The drawing under review shows one solid part. Ordinate dimensions are in mm from its lowest x, y, z. A direction names the side the tool comes from. Coordinates: 2 decimals unless noted, no trailing zeros. Loops run counter-clockwise (first coordinate to the right, second up) from the corner with the lowest first, then second, coordinate; pieces in that order, holes last. Notation, with made-up numbers: (-5.5, 74.25) - (25.5, 74.25) arc R22 ccw to (25.5, 87.25) - close; hole circle Ø4 at (-19, 47.5). An arc over 180 degrees is marked (long way). Answer as a JSON object with one key per item and string values. Group by question number.
Item 1: We need section B-B (x = 8). Give the boundary of the cut face in (y, z).
Item 2: To check wall thickness, follow line 1 (Y direction, x = 42, z = 27.75); line 2 (X direction, y = 20, z = 6.75); line 3 (Y direction, x = 33.5, z = 18.75). State the ranges of each line that lie inside material, in increasing order.
Item 3: We need section A-A (x = 25). Give the boundary of the cut face in (y, z).
Item 4: We need section C-C (y = 25). Give the boundary of the cut face in (x, z), then the cut area to 3 significant figures.
Item 5: Tool access review of the marked faces 1, 2, 3, 4 and 5: name each direction out of +Z, -Z, +X, -X, +Y, -Y from which nothing blocks a thin tool from reaching the whole face with its end or side.
Item 6: Clearance check with flat-ended pins moving along their axes: pin 1 (13 mm diameter, centred on y = 22, z = 14.5, fed in from +X); pin 2 (5.5 mm diameter, centred on x = 23.5, y = 12.5, fed in from +Z); pin 3 (0.8 mm diameter, centred on x = 0.5, y = 25, fed in from +Z); pin 4 (1 mm diameter, centred on x = 42.5, z = 11, fed in from -Y). State where each tip first meets the part, or that it passes through.
Item 7: We need section D-D (z = 22.25). Give the boundary of the cut face in (x, y).
Item 8: Mouldability with a two-part tool opening along X and no side actions: class the marked faces 6, 7 and 8 as released by +X, released by -X, zero draft, split by the parting line, or undercut.
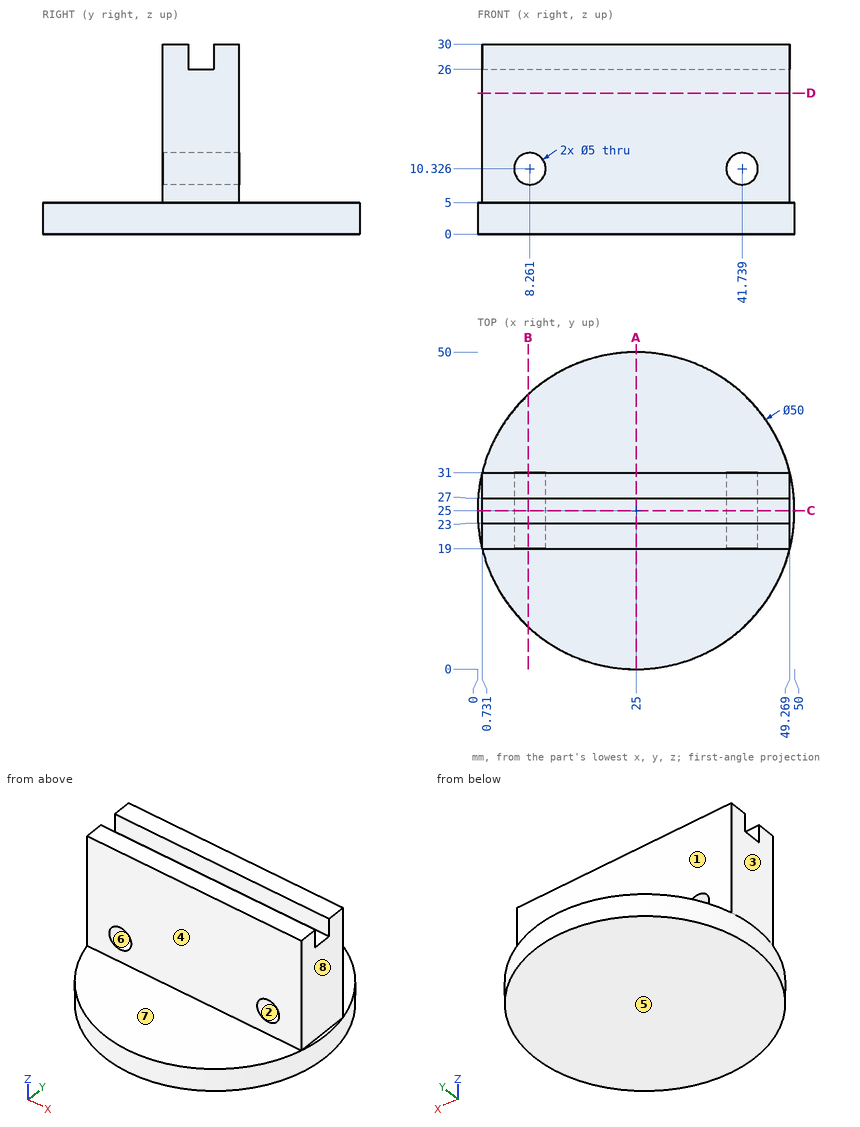
Check sheet entries:
{
 "1": {"outline": "(6.67, 0) - (43.33, 0) - (43.33, 5) - (31, 5) - (31, 7.84) - (19, 7.84) - (19, 5) - (6.67, 5) - close; (19, 12.81) - (31, 12.81) - (31, 30) - (27, 30) - (27, 26) - (23, 26) - (23, 30) - (19, 30) - close"},
 "2": {"line 1": "y = 19 to 23, 27 to 31", "line 2": "x = 0.73 to 49.27", "line 3": "y = 19 to 31"},
 "3": {"outline": "(0, 0) - (50, 0) - (50, 5) - (31, 5) - (31, 30) - (27, 30) - (27, 26) - (23, 26) - (23, 30) - (19, 30) - (19, 5) - (0, 5) - close"},
 "4": {"outline": "(0, 0) - (50, 0) - (50, 5) - (49.27, 5) - (49.27, 26) - (0.73, 26) - (0.73, 5) - (0, 5) - close; hole circle Ø5 at (8.26, 10.33); hole circle Ø5 at (41.74, 10.33)", "area": "1,230 mm2"},
 "5": {"face 1": "+Z, +X, -X, +Y", "face 2": "+Y, -Y", "face 3": "+Z, -X, +Y, -Y", "face 4": "+Z, +X, -X, -Y", "face 5": "-Z, +X, -X, +Y, -Y"},
 "6": {"pin 1": "stops at x = 49.27", "pin 2": "stops at z = 5", "pin 3": "stops at z = 26", "pin 4": "passes through"},
 "7": {"outline": "(0.73, 19) - (49.27, 19) - (49.27, 31) - (0.73, 31) - close"},
 "8": {"face 6": "undercut", "face 7": "zero draft", "face 8": "released by +X"}
}
